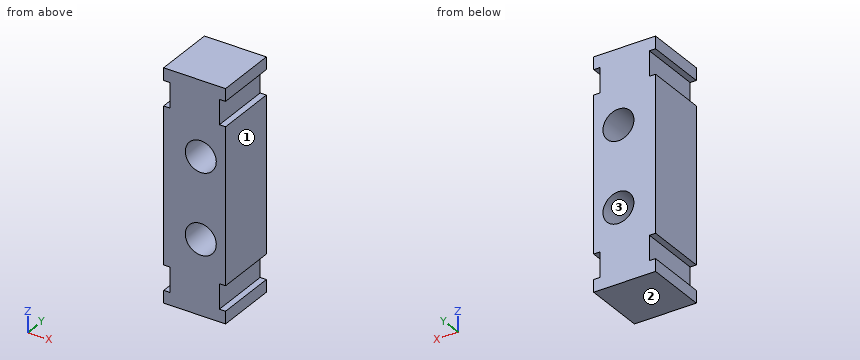
from build123d import *

# Parameters (mm, degrees)
CROQUIS1_W              = 10
CROQUIS1_H              = 10
SALIENTE_EXTRUIR1_DEPTH = 37
CROQUIS2_R              = 2.5
CORTAR_EXTRUIR1_DEPTH   = 39.65229618
CROQUIS4_W              = 1
CROQUIS4_H              = 4
CORTAR_EXTRUIR2_DEPTH   = 39.65229618


with BuildPart() as part:
    # Croquis1 → Saliente-Extruir1 (new body)
    with BuildSketch(Plane.XY):
        Rectangle(CROQUIS1_W, CROQUIS1_H)
    extrude(amount=SALIENTE_EXTRUIR1_DEPTH)

    # Croquis2 → Cortar-Extruir1 (cut, through all)
    with BuildSketch(Plane(origin=(0, 5, 0), x_dir=(1, 0, 0), z_dir=(0, 1, 0))):
        with Locations(Location((1, -12, 0), (0, 0, 270))):
            Circle(CROQUIS2_R)
        with Locations(Location((1, -25, 0), (0, 0, 270))):
            Circle(CROQUIS2_R)
    extrude(amount=-CORTAR_EXTRUIR1_DEPTH, mode=Mode.SUBTRACT)

    # Croquis4 → Cortar-Extruir2 (cut, through all)
    with BuildSketch(Plane(origin=(0, 5, 0), x_dir=(1, 0, 0), z_dir=(0, 1, 0))):
        with Locations((-4.5, -33)):
            Rectangle(CROQUIS4_W, CROQUIS4_H)
        with Locations((4.5, -33)):
            Rectangle(CROQUIS4_W, CROQUIS4_H)
        with Locations((4.5, -4)):
            Rectangle(CROQUIS4_W, CROQUIS4_H)
        with Locations((-4.5, -4)):
            Rectangle(CROQUIS4_W, CROQUIS4_H)
    extrude(amount=-CORTAR_EXTRUIR2_DEPTH, mode=Mode.SUBTRACT)


solid = part.part
Verification items for the finished model (mm, model axes). Face numbers are marked on the shaded views. Coordinates: 2 decimals unless noted, no trailing zeros. Order: outer loops, then holes, each group sorted by start corner. A loop starts at its lowest first (then second) coordinate and runs counter-clockwise, first axis right, second up. Notation, with made-up numbers: M -6,-4 L 15,-4 A32 cw 15,24 Z; hole C 40,-33 d9. An arc over 180 degrees is marked long. Return JSON: item names as keys, results as strings.
1) Cross-section at B-B, the plane x = -1. Record the boundary of the cut face in (y, z), and give its area (3 significant figures).
Answer list:
{"outline": "M -5,0 L 5,0 L 5,10.5 L -5,10.5 Z; M -5,13.5 L 5,13.5 L 5,23.5 L -5,23.5 Z; M -5,26.5 L 5,26.5 L 5,37 L -5,37 Z", "area": "310 mm2"}
2) Cross-section at C-C, the plane y = -0.75. Record the boundary of the cut face in (x, z).
Answer list:
{"outline": "M -5,0 L 5,0 L 5,2 L 4,2 L 4,6 L 5,6 L 5,31 L 4,31 L 4,35 L 5,35 L 5,37 L -5,37 L -5,35 L -4,35 L -4,31 L -5,31 L -5,6 L -4,6 L -4,2 L -5,2 Z; hole C 1,12 d5; hole C 1,25 d5"}
3) Release check for a two-part mould opening along Z. For the marked faces 1, 2 and 3 record: +Z half, -Z half, draft (parallel to the pull), parting line (faces both ways), or undercut.
Answer list:
{"face 1": "draft", "face 2": "-Z half", "face 3": "undercut"}
4) Cross-section at D-D, the plane x = 1. Record the boundary of the cut face in (y, z).
Answer list:
{"outline": "M -5,0 L 5,0 L 5,9.5 L -5,9.5 Z; M -5,14.5 L 5,14.5 L 5,22.5 L -5,22.5 Z; M -5,27.5 L 5,27.5 L 5,37 L -5,37 Z"}
5) Cross-section at A-A, the plane z = 14. Record the boundary of the cut face in (x, y).
Answer list:
{"outline": "M -5,-5 L -0.5,-5 L -0.5,5 L -5,5 Z; M 2.5,-5 L 5,-5 L 5,5 L 2.5,5 Z"}
6) Gauge pin test, flat end, axial feed: pin 1 (1.5 mm diameter, centred on y = -2.5, z = 33, fed in from +X). Record the tip position at first contact, or that the pin passes through.
Answer list:
{"pin 1": "x = 4"}
7) Thickness scan on L1, parallel to Z at x = -4.25, y = -3.25; L2, parallel to Z at x = 3, y = 4; L3, parallel to X at y = -2, z = 12. Record the ranges inside material, lowest first. Write a range as [from, to].
Answer list:
{"L1": "[0, 2], [6, 31], [35, 37]", "L2": "[0, 10.5], [13.5, 23.5], [26.5, 37]", "L3": "[-5, -1.5], [3.5, 5]"}
